Part model, mm, in its own coordinate system. A direction names the side the tool comes from. Give positions to 0.01 mm unless a question says otherwise; leave off trailing zeros. Order: outer loops, then holes, each group sorted by start corner. A loop starts at its lowest first (then second) coordinate and runs counter-clockwise, first axis right, second up. Notation, with made-up numbers: M 48,62 L 99,62 A15 cw 99,70 Z; hole C 43.25,-14 d10. An arc over 180 degrees is marked long. Answer as a JSON object with one key per item and string values.
from build123d import *

# Parameters (mm, degrees)
BOSS_EXTRUDE1_DEPTH     = 15
SKETCH2_R               = 1.5
CUT_EXTRUDE1_DEPTH      = 1
CUT_EXTRUDE1_DEPTH_BACK = 12
CHAMFER1_SIZE           = 0.2
SKETCH4_R               = 1.5
BOSS_EXTRUDE2_DEPTH     = 6.5
CHAMFER2_SIZE           = 0.6


with BuildPart() as part:
    # Sketch1 → Boss-Extrude1 (new body)
    with BuildSketch(Plane.XY):
        Polygon((2.621170222, 0), (1.310585111, 2.27), (-1.310585111, 2.27), (-2.621170222, 0), (-1.310585111, -2.27), (1.310585111, -2.27), align=None)
    extrude(amount=BOSS_EXTRUDE1_DEPTH)

    # Sketch2 → Cut-Extrude1 (cut, two sides)
    with BuildSketch(Plane.XY.offset(15)) as cut_extrude1_sk:
        Circle(SKETCH2_R)
    extrude(amount=CUT_EXTRUDE1_DEPTH, mode=Mode.SUBTRACT)
    extrude(cut_extrude1_sk.sketch, amount=-CUT_EXTRUDE1_DEPTH_BACK, mode=Mode.SUBTRACT)

    # Sketch3 → Cut-Revolve1 (revolve, cut)
    with BuildSketch(Plane(origin=(0, 0, 0), x_dir=(1, 0, 0), z_dir=(0, 1, 0))):
        Polygon((-2.621170222, -15), (-2.271170222, -15), (-2.621170222, -14.8), align=None)
    revolve(axis=Axis((0, 0, 3), (0, 0, 1)), mode=Mode.SUBTRACT)

    # Chamfer1
    chamfer1_edges = [part.edges().sort_by_distance(p)[0] for p in [
        (-1.5, 0, 15),
    ]]
    chamfer(chamfer1_edges, length=CHAMFER1_SIZE)

    # Sketch4 → Boss-Extrude2 (add)
    with BuildSketch(Plane(origin=(0, 0, 0), x_dir=(-1, 0, 0), z_dir=(0, 0, -1))):
        Circle(SKETCH4_R)
    extrude(amount=BOSS_EXTRUDE2_DEPTH)

    # Chamfer2
    chamfer2_edges = [part.edges().sort_by_distance(p)[0] for p in [
        (1.5, 0, -6.5),
    ]]
    chamfer(chamfer2_edges, length=CHAMFER2_SIZE)


solid = part.part
1. Probe line 1 along Y through (x, z) = (0, 7.5); line 2 along Z through (x, y) = (-0.3, 1.7); line 3 along Y through (x, z) = (-0.7, 3.25). List the from-to ranges inside material, lowest first.
Worked answers:
{"line 1": "y = -2.27 to -1.5, 1.5 to 2.27", "line 2": "z = 0 to 15", "line 3": "y = -2.27 to -1.33, 1.33 to 2.27"}
2. Which spindle directions (+Z, -Z, +X, -X, +Y, -Y) get a long thin tool onto all of the face, cutting with end or side? Do faces 4 (the cylindrical face through (-1.5, 0.07, 8.98)), 5 (the flat face through (-1.975, -1.119, 7.395)), 6 (the cylindrical face through (1.5, 0.07, -2.91)). Say none if no direction does.
Worked answers:
{"face 4": "+Z", "face 5": "+Z, -Z, -X, -Y", "face 6": "-Z"}
3. Cut at B-B on z = 1.5. Give the cut face in (x, y), plus the area to 3 significant figures.
Worked answers:
{"outline": "M -2.62,0 L -1.31,-2.27 L 1.31,-2.27 L 2.62,0 L 1.31,2.27 L -1.31,2.27 Z", "area": "17.9 mm^2"}
4. Two-plate mould, pull along X, no slides. Class faces 1 (the flat face through (-1.957, 1.151, 7.395)), 2 (the flat face through (0, 0, 3)), 3 (the flat face through (0, -2.27, 7)): +X half, -X half, draft (parallel to the pull), parting line (faces both ways), or undercut.
Worked answers:
{"face 1": "-X half", "face 2": "undercut", "face 3": "draft"}
5. Cut at A-A on z = 11.75. Give the cut face in (x, y), plus the area to 3 significant figures.
Worked answers:
{"outline": "M -2.62,0 L -1.31,-2.27 L 1.31,-2.27 L 2.62,0 L 1.31,2.27 L -1.31,2.27 Z; hole C 0,0 d3", "area": "10.8 mm^2"}
6. Cut at C-C on z = -2.25. Give the cut face in (x, y).
Worked answers:
{"outline": "C 0,0 d3"}
